CAD build for the part. Positions are in the model's coordinates, mm. Face numbers are marked on the shaded views. A direction names the side the tool comes from. Coordinates: 2 decimals unless noted, no trailing zeros. Order: outer loops, then holes, each group sorted by start corner. A loop starts at its lowest first (then second) coordinate and runs counter-clockwise, first axis right, second up. Notation, with made-up numbers: (30, 36) - (84, 36) arc R9 ccw to (84, 52) - close; hole circle Ø2 at (36.25, -38.75). An arc over 180 degrees is marked (long way). Write each question's results on one line, items separated by ' | '. Start each with the question number.
Q1. Pull direction X, two halves, no side cores. Call the marked faces 5, 6, 7 and 8: released by +X, released by -X, zero draft, split by the parting line, or undercut.
Q2. Which spindle directions (+Z, -Z, +X, -X, +Y, -Y) get a long thin tool onto all of the face, cutting with end or side? Do the marked faces 1, 2, 3 and 4. Say none if no direction does.
Q3. Wall check: probe 1 along Z at (x, y) = (-7, 6.25); probe 2 along Y at (x, z) = (6.5, 23); probe 3 along X at (y, z) = (0.85, 8.5). Give the ranges that are in metal, low to high.
Q4. Band-saw the part on C-C, the plane z = 8.5. Write the cut outline in (x, y), then the cut area to 3 significant figures.
Q5. Band-saw the part on B-B, the plane x = 0. Write the cut outline in (y, z), then the cut area to 3 significant figures.
Q6. Band-saw the part on A-A, the plane y = 6. Write the cut outline in (x, z).
Q7. Pin check, flat tips, straight feed: P1, Ø9, axis at x = 0.5, z = 42.5, coming from the +Y side; P2, Ø6, axis at x = 5, y = 15.5, coming from the -Z side; P3, Ø6.5, axis at x = -0.5, z = -8, coming from the +Y side; P4, Ø12, axis at x = 0, z = 18, coming from the +Y side. Stop position of each tip, or through.
Q8. Band-saw the part on D-D, the plane y = -0.75. Write the cut outline in (x, z), then the cut area to 3 significant figures.
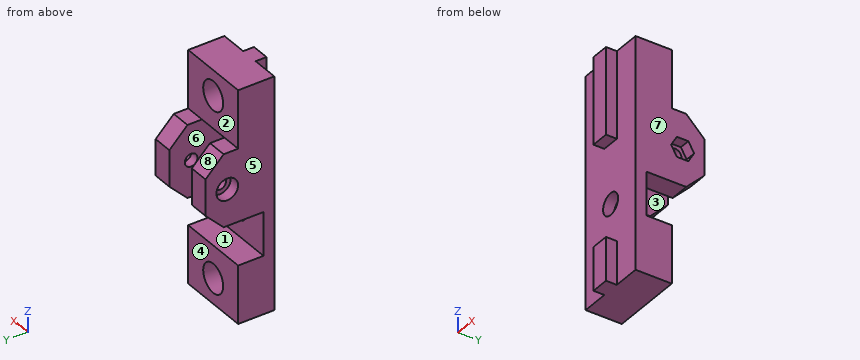
```python
from build123d import *

# Parameters (mm, degrees)
SKETCH1_W               = 20
SKETCH1_H               = 30
BOSS_EXTRUDE1_DEPTH     = 3
SKETCH2_W               = 5
SKETCH2_H               = 12
BOSS_EXTRUDE2_DEPTH     = 3
SKETCH3_R               = 7
SKETCH3_R_2             = 4
BOSS_EXTRUDE3_DEPTH     = 7
SKETCH4_R               = 4
BOSS_EXTRUDE4_DEPTH     = 1
CUT_EXTRUDE1_DEPTH      = 20.339079606
CUT_EXTRUDE1_DEPTH_BACK = 20.339079606
SKETCH5_R               = 3
SKETCH6_R               = 7
SKETCH6_R_2             = 4
BOSS_EXTRUDE6_DEPTH     = 7
SKETCH7_W               = 20
SKETCH7_H               = 3
BOSS_EXTRUDE7_DEPTH     = 19
SKETCH8_W               = 5
SKETCH8_H               = 3
BOSS_EXTRUDE8_DEPTH     = 12
SKETCH10_W              = 5.5
SKETCH10_H              = 20
BOSS_EXTRUDE9_DEPTH     = 16
CUT_EXTRUDE2_DEPTH      = 57.231663678
CUT_EXTRUDE2_DEPTH_BACK = 57.231663678
SKETCH11_R              = 1.75
SKETCH12_R              = 3
SKETCH12_R_2            = 1.75
CUT_EXTRUDE3_DEPTH      = 3
CUT_EXTRUDE4_START      = -3
SKETCH13_R              = 1.75
CUT_EXTRUDE4_DEPTH      = 3
CHAMFER2_SIZE           = 5


with BuildPart() as part:
    # Sketch1 → Boss-Extrude1 (new body)
    with BuildSketch(Plane(origin=(0, 0, 0), x_dir=(1, 0, 0), z_dir=(0, 1, 0))):
        Rectangle(SKETCH1_W, SKETCH1_H)
    boss_extrude1 = extrude(amount=BOSS_EXTRUDE1_DEPTH)

    # Sketch2 → Boss-Extrude2 (add)
    with BuildSketch(Plane.XZ):
        with Locations((0, -9)):
            Rectangle(SKETCH2_W, SKETCH2_H)
    boss_extrude2 = extrude(amount=BOSS_EXTRUDE2_DEPTH)

    # Sketch3 → Boss-Extrude3 (add)
    with BuildSketch(Plane(origin=(0, 3, 0), x_dir=(1, 0, 0), z_dir=(0, 1, 0))):
        with Locations(Location((0, 8, 0), (0, 0, 90))):
            Circle(SKETCH3_R)
        with Locations(Location((0, 8, 0), (0, 0, 270))):
            Circle(SKETCH3_R_2, mode=Mode.SUBTRACT)
    boss_extrude3 = extrude(amount=BOSS_EXTRUDE3_DEPTH)

    # Sketch4 → Boss-Extrude4 (add)
    with BuildSketch(Plane(origin=(0, 3, 0), x_dir=(1, 0, 0), z_dir=(0, 1, 0))):
        with Locations(Location((0, 8, 0), (0, 0, 270))):
            Circle(SKETCH4_R)
    boss_extrude4 = extrude(amount=BOSS_EXTRUDE4_DEPTH)

    # Sketch5 → Cut-Extrude1 (cut, two sides: drawn at the far end of the back side and taken through both)
    with BuildSketch(Plane(origin=(0, 3, 0), x_dir=(1, 0, 0), z_dir=(0, 1, 0)).offset(-CUT_EXTRUDE1_DEPTH_BACK)):
        with Locations(Location((0, -8.5, 0), (0, 0, 90))):
            Circle(SKETCH5_R)
    extrude(amount=CUT_EXTRUDE1_DEPTH + CUT_EXTRUDE1_DEPTH_BACK, mode=Mode.SUBTRACT)

    # Sketch6 → Boss-Extrude6 (add)
    # profile 1 of 2: a face of its own
    with BuildSketch(Plane(origin=(0, 3, 0), x_dir=(1, 0, 0), z_dir=(0, 1, 0))):
        Polygon((0, 15), (-10, 15), (-10, -1), (10, -1), (10, 15), align=None)
        with BuildLine():
            ThreePointArc((7, 8), (-4.949747468, 3.050252532), (0, 15))
            ThreePointArc((0, 15), (4.949747468, 12.949747468), (7, 8))
        make_face(mode=Mode.SUBTRACT)
    # profile 2 of 2: a face of its own
    with BuildSketch(Plane(origin=(0, 3, 0), x_dir=(1, 0, 0), z_dir=(0, 1, 0))):
        with Locations((0, 8)):
            Circle(SKETCH6_R)
        with Locations(Location((0, 8, 0), (0, 0, 270))):
            Circle(SKETCH6_R_2, mode=Mode.SUBTRACT)
    boss_extrude6 = extrude(amount=BOSS_EXTRUDE6_DEPTH)

    # Sketch7 → Boss-Extrude7 (add)
    with BuildSketch(Plane.XY.offset(15)):
        with Locations((0, 1.5)):
            Rectangle(SKETCH7_W, SKETCH7_H)
    extrude(amount=BOSS_EXTRUDE7_DEPTH)

    # Mirror3: Boss-Extrude1, Boss-Extrude2, Boss-Extrude3, Boss-Extrude4, Boss-Extrude6 across plane
    add(boss_extrude1.mirror(Plane.XY.offset(17)))
    add(boss_extrude2.mirror(Plane.XY.offset(17)))
    add(boss_extrude3.mirror(Plane.XY.offset(17)))
    add(boss_extrude4.mirror(Plane.XY.offset(17)))
    add(boss_extrude6.mirror(Plane.XY.offset(17)))

    # Sketch8 → Boss-Extrude8 (add)
    with BuildSketch(Plane(origin=(0, 0, 37), x_dir=(-1, 0, 0), z_dir=(0, 0, -1))):
        with Locations((0, -1.5)):
            Rectangle(SKETCH8_W, SKETCH8_H)
    extrude(amount=BOSS_EXTRUDE8_DEPTH)

    # Sketch10 → Boss-Extrude9 (add)
    with BuildSketch(Plane(origin=(0, 3, 0), x_dir=(1, 0, 0), z_dir=(0, 1, 0))):
        with Locations((-7.25, -23)):
            Rectangle(SKETCH10_W, SKETCH10_H)
        with Locations((7.25, -23)):
            Rectangle(SKETCH10_W, SKETCH10_H)
    extrude(amount=BOSS_EXTRUDE9_DEPTH)

    # Sketch11 → Cut-Extrude2 (cut, two sides: drawn at the far end of the back side and taken through both)
    with BuildSketch(Plane.ZY.offset(10).offset(-CUT_EXTRUDE2_DEPTH_BACK)):
        with Locations((23, 13)):
            Circle(SKETCH11_R)
    extrude(amount=CUT_EXTRUDE2_DEPTH + CUT_EXTRUDE2_DEPTH_BACK, mode=Mode.SUBTRACT)

    # Sketch12 → Cut-Extrude3 (cut)
    with BuildSketch(Plane.ZY.offset(10)):
        with Locations((23, 13)):
            Circle(SKETCH12_R)
        with Locations((23, 13)):
            Circle(SKETCH12_R_2, mode=Mode.SUBTRACT)
    extrude(amount=-CUT_EXTRUDE3_DEPTH, mode=Mode.SUBTRACT)

    # Sketch13 → Cut-Extrude4 (cut)
    with BuildSketch(Plane(origin=(10, 0, 0), x_dir=(0, 0, -1), z_dir=(1, 0, 0)).offset(CUT_EXTRUDE4_START)):
        Polygon((-23, 16.175426481), (-25.75, 14.58771324), (-25.75, 11.41228676), (-23, 9.824573519), (-20.25, 11.41228676), (-20.25, 14.58771324), align=None)
        with Locations((-23, 13)):
            Circle(SKETCH13_R, mode=Mode.SUBTRACT)
    extrude(amount=CUT_EXTRUDE4_DEPTH, mode=Mode.SUBTRACT)

    # Chamfer2
    chamfer2_edges = [part.edges().sort_by_distance(p)[0] for p in [
        (-7.25, 19, 13),
        (-7.25, 19, 33),
        (7.25, 19, 13),
        (7.25, 19, 33),
    ]]
    chamfer(chamfer2_edges, length=CHAMFER2_SIZE)


solid = part.part
```
Results below:
1) face 5: released by -X | face 6: undercut | face 7: released by +X | face 8: zero draft
2) face 1: +X, -X, +Y | face 2: +Z, +X, -X, +Y | face 3: +Y | face 4: -Z, +X, -X, +Y
3) probe 1: z = -15 to 1, 13 to 49 | probe 2: y = 0 to 11.25, 14.75 to 19 | probe 3: x = -10 to -3, 3 to 10
4) outline: (-10, 0) - (-3, 0) - (-3, 3) - (-10, 3) - close; (3, 0) - (10, 0) - (10, 3) - (3, 3) - close | area: 42.0 mm²
5) outline: (-3, -15) - (10, -15) - (10, -12) - (4, -12) - (4, -4) - (10, -4) - (10, 1) - (3, 1) - (3, 5.5) - (0, 5.5) - (0, -3) - (-3, -3) - close; (-3, 25) - (0, 25) - (0, 11.5) - (3, 11.5) - (3, 33) - (10, 33) - (10, 38) - (4, 38) - (4, 46) - (10, 46) - (10, 49) - (-3, 49) - close | area: 410 mm²
6) outline: (-10, -15) - (10, -15) - (10, 1) - (-10, 1) - close; (-10, 13) - (-4.5, 13) - (-4.5, 33) - (4.5, 33) - (4.5, 13) - (10, 13) - (10, 49) - (-10, 49) - close; hole circle Ø8 at (0, -8); hole circle Ø8 at (0, 42)
7) P1: stops at y = 10 | P2: stops at z = 13 | P3: stops at y = 4 | P4: stops at y = 19
8) outline: (-2.5, -15) - (2.5, -15) - (2.5, -3) - (-2.5, -3) - close; (-2.5, 25) - (2.5, 25) - (2.5, 49) - (-2.5, 49) - close | area: 180 mm²
